from build123d import *

# Parameters (mm, degrees)
F0_W     = 20
F0_H     = 10
F0_H_2   = 120
F0_W_2   = 83.6363699974
F0_H_3   = 20
F3_DEPTH = 10
F4_DEPTH = 10


with BuildPart() as f1:
    # F0 (on Right) → F1 (revolve)
    with BuildSketch(Plane.YZ):
        with Locations((-54.3666072938, -174.1780357832)):
            Rectangle(F0_W, F0_H)
        with BuildLine():
            ThreePointArc((-12.7470903483, -159.618054612), (-27.8500467267, -166.7357841949), (-44.3666072938, -169.1780357832))
            Line((-44.3666072938, -169.1780357832), (-44.3666072938, -179.1780357832))
            Line((-44.3666072938, -179.1780357832), (-24.3666072938, -179.1780357832))
            ThreePointArc((-24.3666072938, -179.1780357832), (-19.3081292942, -168.9517504843), (-12.7470903483, -159.618054612))
        make_face()
        with Locations((-14.3666072938, -239.1780357832)):
            Rectangle(F0_W, F0_H_2)
        with Locations((86.542492088, -142.5113668702)):
            Rectangle(F0_W_2, F0_H_3)
        with BuildLine():
            ThreePointArc((44.7243070893, -132.5113668702), (12.9527237019, -139.6280506805), (-12.7470903483, -159.618054612))
            ThreePointArc((-12.7470903483, -159.618054612), (-19.3081292942, -168.9517504843), (-24.3666072938, -179.1780357832))
            Line((-24.3666072938, -179.1780357832), (-4.3666072938, -179.1780357832))
            ThreePointArc((-4.3666072938, -179.1780357832), (16.7912213938, -159.6083850702), (44.7243070893, -152.5113668702))
            Line((44.7243070893, -152.5113668702), (44.7243070893, -132.5113668702))
        make_face()
    revolve(axis=Axis((0, 35.6333935665, -72.5113668702), (0, 1, 0)))

    # F2 (on face) → F3 (cut)
    with BuildSketch(Plane(origin=(0, -4.3666072938, 0), x_dir=(-1, 0, 0), z_dir=(0, 1, 0))):
        with BuildLine():
            ThreePointArc((224.2430593698, -105.5693329389), (122.6869341482, -143.3447013267), (140.7505680979, -250.1825698723))
            ThreePointArc((140.7505680979, -250.1825698723), (196.2990934699, -185.8447013267), (224.2430593698, -105.5693329389))
        make_face()
    extrude(amount=-F3_DEPTH, mode=Mode.SUBTRACT)

    # F2 (on face) → F4 (cut)
    with BuildSketch(Plane(origin=(0, -4.3666072938, 0), x_dir=(-1, 0, 0), z_dir=(0, 1, 0))):
        with BuildLine():
            ThreePointArc((-83.4924912719, -283.2405359411), (0, -299.1780357832), (83.4924912719, -283.2405359411))
            ThreePointArc((83.4924912719, -283.2405359411), (0, -214.1780357832), (-83.4924912719, -283.2405359411))
        make_face()
        with BuildLine():
            ThreePointArc((-224.2430593698, -105.5693329389), (-196.2990934699, -185.8447013267), (-140.7505680979, -250.1825698723))
            ThreePointArc((-140.7505680979, -250.1825698723), (-122.6869341482, -143.3447013267), (-224.2430593698, -105.5693329389))
        make_face()
        with BuildLine():
            ThreePointArc((-140.7505680979, 105.159836132), (-196.2990934699, 40.8219675864), (-224.2430593698, -39.4534008014))
            ThreePointArc((-224.2430593698, -39.4534008014), (-122.6869341482, -1.6780324136), (-140.7505680979, 105.159836132))
        make_face()
        with BuildLine():
            ThreePointArc((140.7505680979, 105.159836132), (122.6869341482, -1.6780324136), (224.2430593698, -39.4534008014))
            ThreePointArc((224.2430593698, -39.4534008014), (196.2990934699, 40.8219675864), (140.7505680979, 105.159836132))
        make_face()
        with BuildLine():
            ThreePointArc((83.4924912719, 138.2178022008), (0, 154.1553020429), (-83.4924912719, 138.2178022008))
            ThreePointArc((-83.4924912719, 138.2178022008), (0, 69.1553020429), (83.4924912719, 138.2178022008))
        make_face()
    extrude(amount=-F4_DEPTH, mode=Mode.SUBTRACT)


solid = f1.part
The model under review builds one solid part; all positions refer to its coordinate system, in mm. A direction names the side the tool comes from. Coordinates: 2 decimals unless noted, no trailing zeros. Order: outer loops, then holes, each group sorted by start corner. A loop starts at its lowest first (then second) coordinate and runs counter-clockwise, first axis right, second up. Notation, with made-up numbers: (5, 6) -> (39, 6) arc R15 ccw to (39, 11) -> close; hole circle Ø5 at (22, 74). An arc over 180 degrees is marked (long way). Answer in a Markdown table with one row per item.
(1) Consider section B-B (x = -174.5). Write out the cut boundary in (y, z), plus the area to 3 significant figures.
Answers:
| item | result |
|---|---|
| outline | (-24.37, -217.17) -> (-14.37, -217.17) -> (-14.37, -103.69) -> (-4.37, -103.69) -> (-4.37, -41.34) -> (-14.37, -41.34) -> (-14.37, 72.15) -> (-24.37, 72.15) -> close |
| area | 3,520 mm² |
(2) Consider section C-C (z = -193). Write out the cut boundary in (x, y), plus the area to 3 significant figures.
Answers:
| item | result |
|---|---|
| outline | (-191.99, -24.37) -> (191.99, -24.37) -> (191.99, -14.37) -> (111.6, -14.37) -> (111.6, -4.37) -> (-111.6, -4.37) -> (-111.6, -14.37) -> (-191.99, -14.37) -> close |
| area | 6,070 mm² |
(3) Machinability: for faces 5 (the flat face through (1, -14.367, 112)), 6 (the cylindrical face through (121.878, -9.297, -144.777)), 7 (the flat face through (47, -24.367, -170)), 8 (the flat face through (1, -14.367, -256)), 9 (the cylindrical face through (-68.085, -16.449, -288.711)), which of the approach directions +Z, -Z, +X, -X, +Y, -Y give a long, thin tool a straight path to every point of the face, cutting with its end or side? Answer none if there is none.
Answers:
| item | result |
|---|---|
| face 5 | +Z, +Y |
| face 6 | +Y |
| face 7 | -Y |
| face 8 | -Z, +Y |
| face 9 | +Y, -Y |
(4) The part is to be moulded in two halves that separate along X. For faces 1 (the cylindrical face through (-32.04, -44.087, -174.252)), 2 (the cylindrical face through (58.82, -54.23, 4.2)), 3 (the flat face through (-16, -64.367, 23)), 4 (the cylindrical face through (-123.52, -9.3, -141.93)), say which applies: +X half, -X half, draft (parallel to the pull), parting line (faces both ways), or undercut.
Answers:
| item | result |
|---|---|
| face 1 | parting line |
| face 2 | undercut |
| face 3 | draft |
| face 4 | undercut |
(5) Wall thickness on line 1 along Z through (x, y) = (0, -52.5); line 2 along Z through (x, y) = (0, 91.5); line 3 along Y through (x, z) = (118.5, 49.5): over which ranges is each line inside the solid? List them lowest first.
Answers:
| item | result |
|---|---|
| line 1 | -179.18 to -169.18, 24.16 to 34.16 |
| line 2 | -152.51 to -132.51, -12.51 to 7.49 |
| line 3 | -24.37 to -14.37 |
(6) Insertion check: pin 1 (2 mm diameter, centred on y = 70.5, z = -34, fed in from -X); pin 2 (1 mm diameter, centred on x = -59.5, y = 81, fed in from -Z); pin 3 (8 mm diameter, centred on y = -13.5, z = -163, fed in from -X). Each pin has a flat end and moves straight along its axis. Give the tip position at first contact, or say it passes through.
Answers:
| item | result |
|---|---|
| pin 1 | x = -70.66 |
| pin 2 | z = -126.54 |
| pin 3 | x = -209.48 |
(7) Consider section D-D (y = 21.5). Write out the cut boundary in (x, z), plus the area to 3 significant figures.
Answers:
| item | result |
|---|---|
| outline | circle Ø169.61 at (0, -72.51); hole circle Ø127.43 at (0, -72.51) |
| area | 9,840 mm² |
(8) Consider section A-A (y = 53.5). Write out the cut boundary in (x, z), plus the area to 3 significant figures.
Answers:
| item | result |
|---|---|
| outline | circle Ø160 at (0, -72.51); hole circle Ø120 at (0, -72.51) |
| area | 8,800 mm² |
